```python
from build123d import *

# Parameters (mm, degrees)
SKETCH1_R                       = 1.7
BOSS_EXTRUDE1_DEPTH             = 3
M3X0_5_TAPPED_HOLE1_D           = 2.5
M3X0_5_TAPPED_HOLE1_DEPTH       = 6.748924226
M3X0_5_TAPPED_HOLE1_CSINK_D     = 3.05
M3X0_5_TAPPED_HOLE1_CSINK_ANGLE = 90
M3X0_5_TAPPED_HOLE1_TIP         = 0.751075774


with BuildPart() as part:
    # Sketch1 → Boss-Extrude1 (new body, symmetric)
    with BuildSketch(Plane.XY):
        with BuildLine():
            Line((38.54163056, 21.04163056), (38.54163056, 27.04163056))
            Line((38.54163056, 27.04163056), (24.04163056, 27.04163056))
            ThreePointArc((24.04163056, 27.04163056), (26.509317815, 25.747655066), (26.848253846, 22.981976969))
            ThreePointArc((26.848253846, 22.981976969), (26.592295747, 22.027653458), (26.528996798, 21.04163056))
            Line((26.528996798, 21.04163056), (38.54163056, 21.04163056))
        make_face()
        with BuildLine():
            ThreePointArc((26.848253846, 22.981976969), (26.509317815, 25.747655066), (24.04163056, 27.04163056))
            ThreePointArc((24.04163056, 27.04163056), (23.503053666, 26.992890449), (22.981976969, 26.848253846))
            ThreePointArc((22.981976969, 26.848253846), (20.97309248, 26.531857751), (19.004373338, 27.04163056))
            Line((19.004373338, 27.04163056), (-19.004373338, 27.04163056))
            ThreePointArc((-19.004373338, 27.04163056), (-20.97309248, 26.531857751), (-22.981976969, 26.848253846))
            ThreePointArc((-22.981976969, 26.848253846), (-23.503053666, 26.992890449), (-24.04163056, 27.04163056))
            ThreePointArc((-24.04163056, 27.04163056), (-26.509317815, 25.747655066), (-26.848253846, 22.981976969))
            ThreePointArc((-26.848253846, 22.981976969), (-25.747655066, 21.573943306), (-24.04163056, 21.04163056))
            Line((-24.04163056, 21.04163056), (26.528996798, 21.04163056))
            ThreePointArc((26.528996798, 21.04163056), (26.592295747, 22.027653458), (26.848253846, 22.981976969))
        make_face()
        with Locations((-24.04163056, 24.04163056)):
            Circle(SKETCH1_R, mode=Mode.SUBTRACT)
        with Locations((24.04163056, 24.04163056)):
            Circle(SKETCH1_R, mode=Mode.SUBTRACT)
        with BuildLine():
            ThreePointArc((22.981976969, 26.848253846), (23.503053666, 26.992890449), (24.04163056, 27.04163056))
            Line((24.04163056, 27.04163056), (19.004373338, 27.04163056))
            ThreePointArc((19.004373338, 27.04163056), (20.97309248, 26.531857751), (22.981976969, 26.848253846))
        make_face()
        with BuildLine():
            ThreePointArc((-22.981976969, 26.848253846), (-20.97309248, 26.531857751), (-19.004373338, 27.04163056))
            Line((-19.004373338, 27.04163056), (-24.04163056, 27.04163056))
            ThreePointArc((-24.04163056, 27.04163056), (-23.503053666, 26.992890449), (-22.981976969, 26.848253846))
        make_face()
    extrude(amount=BOSS_EXTRUDE1_DEPTH, both=True)

    # M3x0.5 Tapped Hole1
    with Locations(Plane(origin=(38.54163056, 24.04163056, 0), x_dir=(0, 0, 1), z_dir=(1, 0, 0))):
        with Locations((0, 0)):
            CounterSinkHole(M3X0_5_TAPPED_HOLE1_D / 2, M3X0_5_TAPPED_HOLE1_CSINK_D / 2, depth=M3X0_5_TAPPED_HOLE1_DEPTH, counter_sink_angle=M3X0_5_TAPPED_HOLE1_CSINK_ANGLE)
            with Locations((0, 0, -(M3X0_5_TAPPED_HOLE1_DEPTH + M3X0_5_TAPPED_HOLE1_TIP / 2))):  # 118° drill point
                Cone(0, M3X0_5_TAPPED_HOLE1_D / 2, M3X0_5_TAPPED_HOLE1_TIP, mode=Mode.SUBTRACT)


solid = part.part
```
Work out the finished part from the listing and answer in its coordinate system (mm). Give positions to 0.01 mm unless a question says otherwise; leave off trailing zeros. Loops run counter-clockwise (first coordinate to the right, second up) from the corner with the lowest first, then second, coordinate; pieces in that order, holes last. Notation, with made-up numbers: (10, -24) -> (61, -24) arc R21 ccw to (61, 15) -> close; hole circle Ø1 at (-2, -33). An arc over 180 degrees is marked (long way). One line per question, with ' | ' between items. Start each with the question number.
1) Determine the mould class of faces 1 (the face through (34.98, 22.8, 0.16)), 2 (the face through (-27.04, 24.11, 0.04)), 3 (the face through (38.542, 22.7, 1.4)) for opening direction Y: +Y half, -Y half, draft (parallel to the pull), parting line (faces both ways), or undercut.
2) Section A-A, the plane z = -2.1 is taken. Determine the outline of the cut face in (x, y).
3) Straight lines are drawn through the part: L1, parallel to Y at x = 24, z = 2.2; L2, parallel to X at y = 24.8, z = -1.95; L3, parallel to X at y = 22.6, z = 0.7. For each, find the intervals that lie inside material, in ascending order.
Resolved:
1) face 1: undercut | face 2: parting line | face 3: draft
2) outline: (-24.04, 21.04) -> (38.54, 21.04) -> (38.54, 27.04) -> (-24.04, 27.04) arc R3 ccw to start; hole circle Ø3.4 at (-24.04, 24.04); hole circle Ø3.4 at (24.04, 24.04)
3) L1: 21.04 to 22.34, 25.74 to 27.04 | L2: -26.94 to -25.56, -22.52 to 22.52, 25.56 to 38.54 | L3: -26.67 to -24.94, -23.14 to 23.14, 24.94 to 38.54
